The drawing under review shows one solid part. Ordinate dimensions are in mm from its lowest x, y, z. A direction names the side the tool comes from. Give positions to 0.01 mm unless a question says otherwise; leave off trailing zeros. Loops run counter-clockwise (first coordinate to the right, second up) from the corner with the lowest first, then second, coordinate; pieces in that order, holes last. Notation, with made-up numbers: (-21, -29.75) - (28, -29.75) arc R33 cw to (28, 5.25) - close; hole circle Ø9 at (0.25, 24.5). An arc over 180 degrees is marked (long way). Return JSON: item names as keys, results as strings. Group by question number.
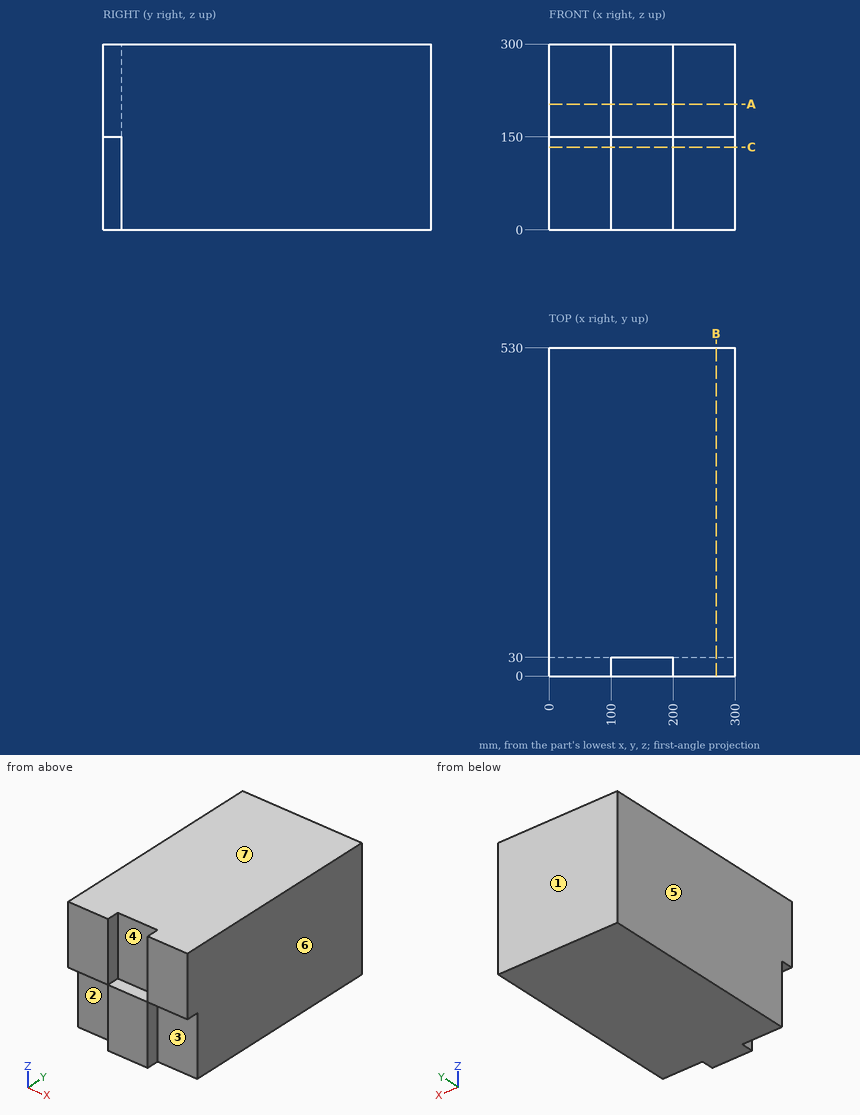
1) We need section A-A, the plane z = 203. Write out the cut boundary in (x, y), plus the area to 3 significant figures.
2) To check wall thickness, follow line 1 (Y direction, x = 48, z = 50). State the ranges of the line that lie inside material, in increasing order.
3) Draft analysis for pull direction X (two halves, no side actions). For the marked faces 4, 5, 6 and 7, state which applies: +X half, -X half, draft (parallel to the pull), parting line (faces both ways), or undercut.
4) Tool access review of the marked faces 1, 2 and 3: name each direction out of +Z, -Z, +X, -X, +Y, -Y from which nothing blocks a thin tool from reaching the whole face with its end or side.
5) For pin 1 Ø1 at (x, z) = (207.5, 256.5) entering from -Y; pin 2 Ø15 at (x, y) = (137.5, 8) entering from +Z; pin 3 Ø15 at (y, z) = (8.5, 84) entering from -X; pin 4 Ø15 at (y, z) = (12, 44.5) entering from +X, all flat-tipped, find the tip position at first contact; note any pin that passes through.
6) We need section C-C, the plane z = 133.5. Write out the cut boundary in (x, y), plus the area to 3 significant figures.
7) We need section B-B, the plane x = 269.5. Write out the cut boundary in (y, z), plus the area to 4 significant figures.
Findings:
{
 "1": {"outline": "(0, 0) - (100, 0) - (100, 30) - (200, 30) - (200, 0) - (300, 0) - (300, 530) - (0, 530) - close", "area": "156,000 mm^2"},
 "2": {"line 1": "y = 30 to 530"},
 "3": {"face 4": "undercut", "face 5": "-X half", "face 6": "+X half", "face 7": "draft"},
 "4": {"face 1": "+Z, -Z, +X, -X, +Y", "face 2": "-Z, -X, -Y", "face 3": "-Z, +X, -Y"},
 "5": {"pin 1": "stops at y = 0", "pin 2": "stops at z = 150", "pin 3": "stops at x = 100", "pin 4": "stops at x = 200"},
 "6": {"outline": "(0, 30) - (100, 30) - (100, 0) - (200, 0) - (200, 30) - (300, 30) - (300, 530) - (0, 530) - close", "area": "153,000 mm^2"},
 "7": {"outline": "(0, 150) - (30, 150) - (30, 0) - (530, 0) - (530, 300) - (0, 300) - close", "area": "154,500 mm^2"}
}
